Design review of the part built by this model. Coordinates are the model's own, in mm. Face numbers are marked on the shaded views. A direction names the side the tool comes from. Give positions to 0.01 mm unless a question says otherwise; leave off trailing zeros. Loops run counter-clockwise (first coordinate to the right, second up) from the corner with the lowest first, then second, coordinate; pieces in that order, holes last. Notation, with made-up numbers: M 12.25,78.25 L 18.25,78.25 A21 ccw 18.25,103.25 Z; hole C 26,-20.75 d5. An arc over 180 degrees is marked long. Use a Markdown table: item, result. Add a question column.
(1) Add section A-A, the plane x = 68.5. Give the boundary of the cut face in (y, z).
(2) Insertion check: pin 1 Ø1.5 at (y, z) = (37.5, 0) entering from +X (3 decimals); pin 2 Ø4 at (x, y) = (15.5, 3.5) entering from +Z; pin 3 Ø12 at (y, z) = (15, 49.5) entering from -X. Each pin has a flat end and moves straight along its axis. Give the tip position at first contact, or say it passes through.
(3) Add section B-B, the plane y = 47.5. Give the boundary of the cut face in (x, z) (3 decimals).
(4) For probe 1 along Y at (x, z) = (-3.5, 18.5); probe 2 along X at (y, z) = (20.5, 11) (3 decimals); probe 3 along X at (y, z) = (-32, 4.5) (3 decimals), list the stretches that pass through material, from the lowest coordinate up.
(5) For the marked faces 1, 2 and 3, list the 3-axis set-ups (+Z, -Z, +X, -X, +Y, -Y) from which the entire face can be reached by the end or side of a thin tool; tool diameter is ignored.
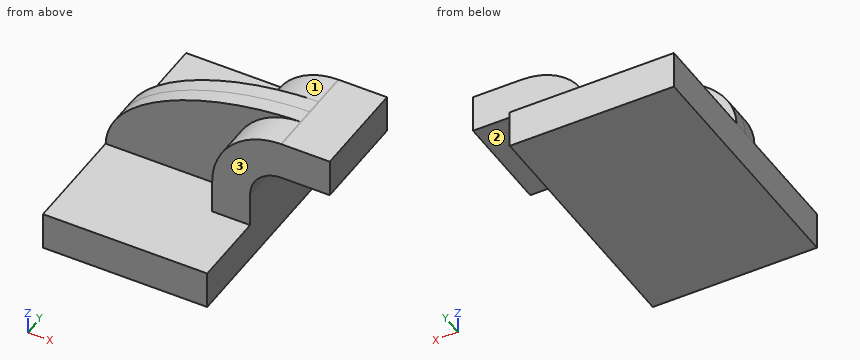
```python
from build123d import *

# Parameters (mm, degrees)
F1_DEPTH = 63.5
F2_DEPTH = 7.9375
F0_W     = 20.994958
F0_H     = 19.05
F3_DEPTH = 25.4


with BuildPart() as f1:
    # F0 (on Front) → F1 (new body, symmetric)
    with BuildSketch(Plane.XZ):
        Polygon((22.225, 9.525), (-41.275, 9.525), (-41.275, -9.525), (41.275, -9.525), (41.275, 9.525), align=None)
    extrude(amount=F1_DEPTH, both=True)

    # F0 (on Front) → F2 (join, symmetric)
    with BuildSketch(Plane.XZ):
        with BuildLine():
            add(Edge.make_bspline(
                [(-41.275, 9.525), (-40.245121, 41.951919), (14.464107, 61.571726), (56.686629, 61.922126)],
                knots=[0, 0, 0, 0, 111.097679, 111.097679, 111.097679, 111.097679], degree=3))
            Line((-41.275, 9.525), (22.225, 9.525))
            Line((22.225, 9.525), (22.225, 27.0002))
            ThreePointArc((22.225, 27.0002), (32.291009, 51.531531), (56.686629, 61.922126))
        make_face()
    extrude(amount=F2_DEPTH, both=True)

    # F0 (on Front) → F3 (join, symmetric)
    with BuildSketch(Plane.XZ):
        with Locations((70.822479, 52.4002)):
            Rectangle(F0_W, F0_H)
        with BuildLine():
            Line((22.225, 27.0002), (22.225, 9.525))
            Line((22.225, 9.525), (41.275, 9.525))
            Line((41.275, 9.525), (41.275, 27.0002))
            ThreePointArc((41.275, 27.0002), (45.92468, 38.22552), (57.15, 42.8752))
            Line((57.15, 42.8752), (60.325, 42.8752))
            Line((60.325, 42.8752), (60.325, 61.9252))
            Line((60.325, 61.9252), (57.15, 61.9252))
            add(Edge.make_bspline(
                [(56.686629, 61.922126), (56.841254, 61.923409), (56.995713, 61.924434), (57.15, 61.9252)],
                knots=[111.097679, 111.097679, 111.097679, 111.097679, 111.504536, 111.504536, 111.504536, 111.504536], degree=3))
            ThreePointArc((56.686629, 61.922126), (32.291009, 51.531531), (22.225, 27.0002))
        make_face()
    extrude(amount=F3_DEPTH, both=True)


solid = f1.part
```
Established:
| question | item | result |
|---|---|---|
| 1 | outline | M -25.4,42.88 L 25.4,42.88 L 25.4,61.93 L -25.4,61.93 Z |
| 2 | pin 1 | x = 41.275 |
| 2 | pin 2 | z = 56.68 |
| 2 | pin 3 | x = 26.37 |
| 3 | outline | M -41.275,-9.525 L 41.275,-9.525 L 41.275,9.525 L -41.275,9.525 Z |
| 4 | probe 1 | -7.94 to 7.94 |
| 4 | probe 2 | 22.225 to 41.275 |
| 4 | probe 3 | -41.275 to 41.275 |
| 5 | face 1 | +Z, -X, +Y |
| 5 | face 2 | -Z, +X, +Y, -Y |
| 5 | face 3 | +Z, +X, -X, -Y |
